The figure shows three views and two pictorial views of one solid part (mm, origin at its lowest corner). Answer the questions. A direction names the side the tool comes from. Coordinates: 2 decimals unless noted, no trailing zeros. Write each loop counter-clockwise with the first axis right and the second up, starting at its lowest first coordinate (ties: lowest second). Pieces come first, ordered by that corner, then holes.
Item 1: Section C-C (y = 82) is taken. Give the vertices of the cut face in (x, z), then the cut area to 3 significant figures.
Item 2: A tool of negligible diameter and unlimited length cuts with its end or side. For the marked faces 1 and 2, from which of +Z, -Z, +X, -X, +Y, -Y can it reach the whole face along a straight path? Write none if from no direction.
Item 3: Section D-D (y = 54.5) is taken. Give the vertices of the cut face in (x, z).
Item 4: Section A-A (y = 139.5) is taken. Give the vertices of the cut face in (x, z).
Item 5: Straight lines are drawn through the part: probe 1 along Z at (x, y) = (55, 116); probe 2 along X at (y, z) = (143.5, 56); probe 3 along Z at (x, y) = (55, 122). For each, find the intervals that lie inside material, in ascending order.
Item 6: Each of these flat-tipped pins is pushed along its axis until it touches: P1, Ø1.5, axis at x = 73.5, y = 105.5, coming from the -Z side; P2, Ø3, axis at y = 106.5, z = 110.5, coming from the +X side; P3, Ø8, axis at x = 79, y = 87.5, coming from the -Z side. Where does it stop, or does it pass through?
Item 7: Section B-B (z = 116.5) is taken. Give the vertices of the cut face in (x, y), then the cut area to 3 significant figures.
Item 8: Determine the mould class of the marked faces 3, 4 and 5 for opening direction Z: released by +Z, released by -Z, zero draft, split by the parting line, or undercut.
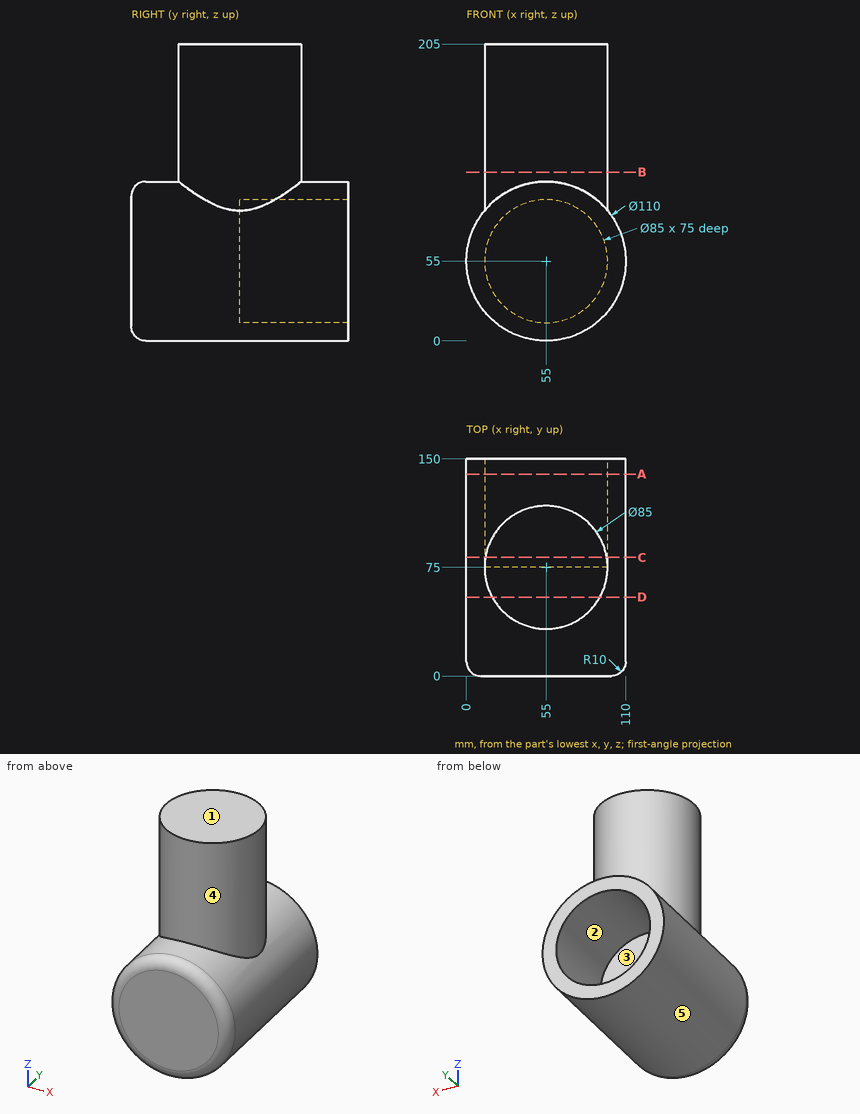
Established:
1. outline: (13.08, 90.61) arc R55 ccw (long way) to (96.92, 90.61) - (96.92, 205) - (13.08, 205) - close; hole circle Ø85 at (55, 55)
1. area: 12,300 mm2
2. face 1: +Z, +X, -X, +Y, -Y
2. face 2: +Y
3. outline: (17.77, 95.48) arc R55 ccw (long way) to (92.23, 95.48) - (92.23, 205) - (17.77, 205) - close
4. outline: circle Ø110 at (55, 55); hole circle Ø85 at (55, 55)
5. probe 1: z = 0 to 12.5, 97.5 to 205
5. probe 2: x = 0.01 to 12.51, 97.49 to 109.99
5. probe 3: z = 0 to 12.5, 97.5 to 110
6. P1: stops at z = 2.94
6. P2: stops at x = 85.1
6. P3: stops at z = 3.77
7. outline: circle Ø85 at (55, 75)
7. area: 5,670 mm2
8. face 3: undercut
8. face 4: zero draft
8. face 5: split by the parting line
